from build123d import *

# Parameters (mm, degrees)
SKETCH1_W           = 43
SKETCH1_H           = 40
BOSS_EXTRUDE1_DEPTH = 5
SKETCH2_W           = 13
SKETCH2_H           = 2
SKETCH2_W_2         = 17.5
SKETCH2_W_3         = 2.5
SKETCH2_H_2         = 10
BOSS_EXTRUDE3_DEPTH = 8
BOSS_EXTRUDE4_DEPTH = 15
SKETCH4_R           = 1.5
CUT_EXTRUDE1_DEPTH  = 65
SKETCH6_R           = 1.5
CUT_EXTRUDE2_DEPTH  = 10
SKETCH7_R           = 6.5
CUT_EXTRUDE3_DEPTH  = 20
SKETCH8_W           = 15
SKETCH8_H           = 20
CUT_EXTRUDE4_DEPTH  = 5
FILLET1_R           = 1
FILLET2_R           = 1


with BuildPart() as part:
    # Sketch1 → Boss-Extrude1 (new body)
    with BuildSketch(Plane.XY):
        with Locations((75.504805995, -8.785410368)):
            Rectangle(SKETCH1_W, SKETCH1_H)
    extrude(amount=BOSS_EXTRUDE1_DEPTH)

    # Sketch2 → Boss-Extrude3 (add)
    with BuildSketch(Plane(origin=(0, 0, 0), x_dir=(-1, 0, 0), z_dir=(0, 0, -1))):
        with Locations((-79.004805995, -0.485410368)):
            Rectangle(SKETCH2_W, SKETCH2_H)
        with Locations((-76.754805995, -16.985410368)):
            Rectangle(SKETCH2_W_2, SKETCH2_H)
        with Locations((-66.754805995, -9.285410368)):
            Rectangle(SKETCH2_W_3, SKETCH2_H_2)
    extrude(amount=BOSS_EXTRUDE3_DEPTH)

    # Sketch3 → Boss-Extrude4 (add)
    with BuildSketch(Plane(origin=(0, 0, 0), x_dir=(-1, 0, 0), z_dir=(0, 0, -1))):
        Polygon((-54.004805995, 11.214589632), (-97.004805995, 11.214589632), (-97.004805995, -28.785410368), (-54.004805995, -28.785410368), (-54.004805995, -25.285410368), (-93.504805995, -25.285410368), (-93.504805995, 7.714589632), (-54.004805995, 7.714589632), align=None)
    extrude(amount=BOSS_EXTRUDE4_DEPTH)

    # Sketch4 → Cut-Extrude1 (cut)
    with BuildSketch(Plane(origin=(0, 11.214589632, 0), x_dir=(1, 0, 0), z_dir=(0, 1, 0))):
        with Locations(Location((83.004805995, 5, 0), (0, 0, 180))):
            Circle(SKETCH4_R)
    extrude(amount=-CUT_EXTRUDE1_DEPTH, mode=Mode.SUBTRACT)

    # Sketch6 → Cut-Extrude2 (cut)
    with BuildSketch(Plane.XZ.offset(28.785410368)):
        with Locations((60.004805995, -5)):
            Circle(SKETCH6_R)
    extrude(amount=-CUT_EXTRUDE2_DEPTH, mode=Mode.SUBTRACT)

    # Sketch7 → Cut-Extrude3 (cut)
    with BuildSketch(Plane.XY.offset(5)):
        with Locations((76.004805995, -8.785410368)):
            Circle(SKETCH7_R)
    extrude(amount=-CUT_EXTRUDE3_DEPTH, mode=Mode.SUBTRACT)

    # Sketch8 → Cut-Extrude4 (cut)
    with BuildSketch(Plane(origin=(97.004805995, 0, 0), x_dir=(0, 0, -1), z_dir=(1, 0, 0))):
        with Locations((7.5, -8.785410368)):
            Rectangle(SKETCH8_W, SKETCH8_H)
    extrude(amount=-CUT_EXTRUDE4_DEPTH, mode=Mode.SUBTRACT)

    # Fillet1
    fillet1_edges = [part.edges().sort_by_distance(p)[0] for p in [
        (54.004805995, 11.214589632, -5),
        (54.004805995, -8.785410368, 5),
        (75.504805995, -28.785410368, 5),
        (97.004805995, -28.785410368, -5),
        (97.004805995, -8.785410368, 5),
        (75.504805995, 11.214589632, 5),
        (97.004805995, 11.214589632, -5),
        (97.004805995, 6.214589632, -15),
        (75.504805995, 11.214589632, -15),
    ]]
    fillet(fillet1_edges, radius=FILLET1_R)

    # Fillet2
    fillet2_edges = [part.edges().sort_by_distance(p)[0] for p in [
        (94.754805995, 1.214589632, -15),
        (95.254805995, -18.785410368, -15),
        (97.004805995, -8.785410368, 0),
        (97.004805995, -18.785410368, -7.5),
        (97.004805995, 1.214589632, -7),
        (96.711912776, 1.214589632, -14.707106781),
    ]]
    fillet(fillet2_edges, radius=FILLET2_R)


solid = part.part
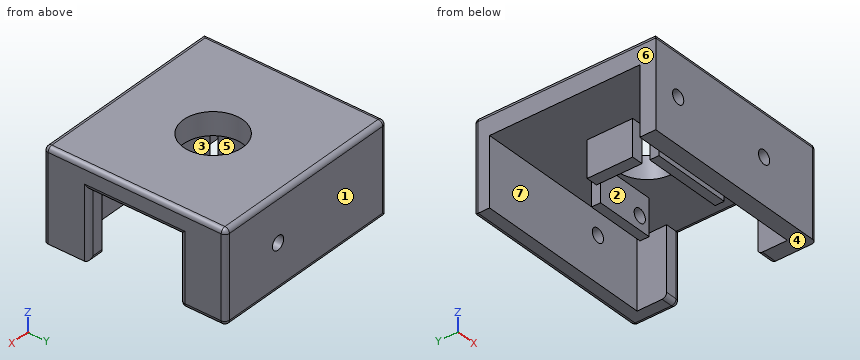
Input: part model. Units: mm. Frame: model coordinates. Face numbers are marked on the shaded views. A direction names the side the tool comes from. Round coordinates to 2 decimals unless told otherwise and drop trailing zeros. Loops run counter-clockwise (first coordinate to the right, second up) from the corner with the lowest first, then second, coordinate; pieces in that order, holes last. Notation, with made-up numbers: (35.25, 82) -> (58.25, 82) arc R20 cw to (58.25, 90) -> close; hole circle Ø2 at (-18.5, -21). An arc over 180 degrees is marked (long way). Answer as a JSON object with one key per item and string values. Group by question number.
1) Section query A-A on z = -1.25. State how many separate pieces and enclosed holes the cut face has, plus the area to 3 significant figures.
2) Section query B-B on z = -11.5. Output: boundary loops of the cut face in (x, y).
3) Ray query, L1, parallel to Y at x = 74.5, z = -7; L2, parallel to Y at x = 59, z = -6.75; L3, parallel to Y at x = 94, z = -8.5. Return the intervals inside material, ascending.
4) Reachability of the marked faces 5, 6 and 7 from +Z, -Z, +X, -X, +Y, -Y: full face, straight path, thin tool, end or side. Return the list, or none.
5) Section query D-D on x = 78. Output: boundary loops of the cut face in (y, z), plus the area to 3 significant figures.
6) Section query C-C on x = 67. Output: boundary loops of the cut face in (y, z), plus the area to 3 significant figures.
7) Pin query (flat end, axial travel): pin 1 (0.8 mm diameter, centred on x = 66, y = -9, fed in from -Z); pin 2 (3 mm diameter, centred on x = 89.5, y = -14.5, fed in from -Z); pin 3 (2 mm diameter, centred on y = -21.5, z = -4.5, fed in from -X). Return the tip coordinate at first contact, or that it passes through.
8) Draft query along Y for the marked faces 1, 2, 3 and 4. Return one class per face: +Y half, -Y half, draft (parallel to the pull), parting line (faces both ways), or undercut.
Reply:
{
 "1": {"separate pieces": "5", "enclosed holes": "0", "area": "431 mm2"},
 "2": {"outline": "(54, -28.79) -> (96, -28.79) arc R1 ccw to (97, -27.79) -> (97, -19.79) arc R1 ccw to (96, -18.79) -> (93.5, -18.79) -> (93.5, -25.29) -> (54, -25.29) -> close; (54, 7.71) -> (93.5, 7.71) -> (93.5, 1.21) -> (96, 1.21) arc R1 ccw to (97, 2.21) -> (97, 10.21) arc R1 ccw to (96, 11.21) -> (55, 11.21) arc R1 ccw to (54, 10.21) -> close"},
 "3": {"L1": "y = -28.79 to -25.29, -17.99 to -15.99, -1.49 to 0.51, 7.71 to 11.21", "L2": "y = -28.79 to -25.29, 7.71 to 11.21", "L3": "y = -28.79 to -18.79, 1.21 to 11.21"},
 "4": {"face 5": "-Z, +X", "face 6": "+Z, -Z, -X, +Y, -Y", "face 7": "-Z, -X"},
 "5": {"outline": "(-28.79, -15) -> (-25.29, -15) -> (-25.29, 0) -> (-17.99, 0) -> (-17.99, -8) -> (-15.99, -8) -> (-15.99, 0) -> (-14.97, 0) -> (-14.97, 5) -> (-27.79, 5) arc R1 ccw to (-28.79, 4) -> close; (-2.6, 0) -> (-1.49, 0) -> (-1.49, -8) -> (0.51, -8) -> (0.51, 0) -> (7.71, 0) -> (7.71, -15) -> (10.21, -15) arc R1 ccw to (11.21, -14) -> (11.21, 4) arc R1 ccw to (10.21, 5) -> (-2.6, 5) -> close", "area": "274 mm2"},
 "6": {"outline": "(-28.79, -15) -> (-25.29, -15) -> (-25.29, 0) -> (-14.29, 0) -> (-14.29, -8) -> (-4.29, -8) -> (-4.29, 0) -> (7.71, 0) -> (7.71, -15) -> (10.21, -15) arc R1 ccw to (11.21, -14) -> (11.21, 4) arc R1 ccw to (10.21, 5) -> (-27.79, 5) arc R1 ccw to (-28.79, 4) -> close", "area": "384 mm2"},
 "7": {"pin 1": "stops at z = -8", "pin 2": "stops at z = 0", "pin 3": "stops at x = 93.5"},
 "8": {"face 1": "+Y half", "face 2": "undercut", "face 3": "undercut", "face 4": "draft"}
}
